Build history of the part. All positions in model axes, mm. Face numbers are marked on the shaded views. A direction names the side the tool comes from. Give positions to 0.01 mm unless a question says otherwise; leave off trailing zeros. Write each loop counter-clockwise with the first axis right and the second up, starting at its lowest first coordinate (ties: lowest second). Pieces come first, ordered by that corner, then holes. Notation, with made-up numbers: (79.25, 2.25) -> (84.25, 2.25) arc R14 ccw to (84.25, 12.25) -> close; hole circle Ø3 at (15, 44.5). An arc over 180 degrees is marked (long way). Put each result on its own line as item: value.
from build123d import *

# Parameters (mm, degrees)
BOSS_EXTRUDE1_DEPTH      = 7
SKETCH2_R                = 2.05
CUT_EXTRUDE1_DEPTH       = 210.034905978
CUT_EXTRUDE2_DEPTH       = 4
BOSS_EXTRUDE8_DEPTH      = 7
BOSS_EXTRUDE8_DEPTH_BACK = 1
BOSS_EXTRUDE9_DEPTH      = 8
SKETCH22_R               = 2
CUT_EXTRUDE3_DEPTH       = 211.072825271
CUT_EXTRUDE4_DEPTH       = 4
CHAMFER1_SIZE            = 0.5
CHAMFER2_SIZE            = 0.5
CHAMFER3_SIZE            = 4


with BuildPart() as part:
    # Sketch1 → Boss-Extrude1 (new body)
    with BuildSketch(Plane.XY):
        Polygon((-86.168640192, 66.168375393), (-46.796854981, 26.9381166), (-46.864915159, 16.542640687), (-68.155605804, 16.542640687), (-75.083809034, 4.542640687), (-88.767010414, 4.542640687), (-95.695213644, 16.542640687), (-127.7, 16.542640687), (-127.7, 21.829570993), (-140.170429007, 34.3), (-155.457359313, 34.3), (-155.457359313, 76.089816153), (-167.457359313, 83.018019384), (-167.457359313, 96.701220763), (-155.457359313, 103.629423994), (-155.457359313, 124.918472329), (-145.062341245, 124.850415149), (-105.649268389, 85.614252867), (-92.265224659, 89.200496576), (-82.589740175, 79.525012092), align=None)
    extrude(amount=-BOSS_EXTRUDE1_DEPTH)

    # Sketch2 → Cut-Extrude1 (cut, through all)
    with BuildSketch(Plane(origin=(0, 0, -7), x_dir=(-1, 0, 0), z_dir=(0, 0, -1))):
        with Locations((82.1403802, 10.392640687)):
            Circle(SKETCH2_R)
        with Locations((91.564057064, 80.226179394)):
            Circle(SKETCH2_R)
        with Locations((161.607359313, 89.8596198)):
            Circle(SKETCH2_R)
    extrude(amount=-CUT_EXTRUDE1_DEPTH, mode=Mode.SUBTRACT)

    # Sketch3 → Cut-Extrude2 (cut)
    with BuildSketch(Plane.XY):
        Polygon((-158.61957167, 88.1346198), (-158.61957167, 91.5846198), (-161.607359313, 93.3096198), (-164.595146956, 91.5846198), (-164.595146956, 88.1346198), (-161.607359313, 86.4096198), align=None)
        Polygon((-88.231612963, 81.1191051), (-90.671131358, 83.558623495), (-94.003575459, 82.665697789), (-94.896501165, 79.333253689), (-92.456982769, 76.893735294), (-89.124538669, 77.786660999), align=None)
        Polygon((-80.4153802, 7.404853044), (-78.6903802, 10.392640687), (-80.4153802, 13.38042833), (-83.8653802, 13.38042833), (-85.5903802, 10.392640687), (-83.8653802, 7.404853044), align=None)
    extrude(amount=-CUT_EXTRUDE2_DEPTH, mode=Mode.SUBTRACT)

    # Sketch19 → Boss-Extrude8 (add, two sides: drawn at the far end of the back side and taken through both)
    with BuildSketch(Plane(origin=(0, 0, -7), x_dir=(-1, 0, 0), z_dir=(0, 0, -1)).offset(-BOSS_EXTRUDE8_DEPTH_BACK)):
        Polygon((46.864915159, 16.542640687), (46.796854981, 26.9381166), (145.062341245, 124.850415149), (155.457359313, 124.918472329), (155.457359313, 34.3), (140.170429007, 34.3), (127.7, 21.829570993), (127.7, 16.542640687), align=None)
    extrude(amount=BOSS_EXTRUDE8_DEPTH + BOSS_EXTRUDE8_DEPTH_BACK)

    # Sketch20 → Boss-Extrude9 (add)
    with BuildSketch(Plane(origin=(0, 0, -14), x_dir=(-1, 0, 0), z_dir=(0, 0, -1))):
        Polygon((127.7, 16.542640687), (107.164334943, 16.542640687), (71.827840432, 51.879135198), (119.997668017, 99.875829855), (155.457359313, 64.416138559), (155.457359313, 34.3), (140.170429007, 34.3), (127.7, 21.829570993), align=None)
    extrude(amount=BOSS_EXTRUDE9_DEPTH)

    # Sketch22 → Cut-Extrude3 (cut, through all)
    with BuildSketch(Plane(origin=(0, 0, -22), x_dir=(-1, 0, 0), z_dir=(0, 0, -1))):
        with Locations((100.752632712, 46.288866697)):
            Circle(SKETCH22_R)
        with Locations((125.501370054, 71.037604039)):
            Circle(SKETCH22_R)
    extrude(amount=-CUT_EXTRUDE3_DEPTH, mode=Mode.SUBTRACT)

    # Sketch23 → Cut-Extrude4 (cut)
    with BuildSketch(Plane.XY):
        Polygon((-125.501370054, 74.487604039), (-128.489157697, 72.762604039), (-128.489157697, 69.312604039), (-125.501370054, 67.587604039), (-122.513582411, 69.312604039), (-122.513582411, 72.762604039), align=None)
        Polygon((-104.202632712, 46.288866697), (-102.477632712, 43.301079054), (-99.027632712, 43.301079054), (-97.302632712, 46.288866697), (-99.027632712, 49.27665434), (-102.477632712, 49.27665434), align=None)
    extrude(amount=-CUT_EXTRUDE4_DEPTH, mode=Mode.SUBTRACT)

    # Chamfer1
    chamfer1_edges = [part.edges().sort_by_distance(p)[0] for p in [
        (-160.113465491, 87.2721198, 0),
        (-158.61957167, 89.8596198, 0),
        (-160.113465491, 92.4471198, 0),
        (-163.101253134, 92.4471198, 0),
        (-164.595146956, 89.8596198, 0),
        (-163.101253134, 87.2721198, 0),
        (-88.678075816, 79.45288305, 0),
        (-89.451372161, 82.338864297, 0),
        (-92.337353409, 83.112160642, 0),
        (-94.450038312, 80.999475739, 0),
        (-93.676741967, 78.113494491, 0),
        (-90.790760719, 77.340198146, 0),
        (-82.1403802, 7.404853044, 0),
        (-79.5528802, 8.898746866, 0),
        (-79.5528802, 11.886534509, 0),
        (-82.1403802, 13.38042833, 0),
        (-84.7278802, 11.886534509, 0),
        (-84.7278802, 8.898746866, 0),
    ]]
    chamfer(chamfer1_edges, length=CHAMFER1_SIZE)

    # Chamfer2
    chamfer2_edges = [part.edges().sort_by_distance(p)[0] for p in [
        (-124.007476232, 73.625104039, 0),
        (-126.995263875, 73.625104039, 0),
        (-128.489157697, 71.037604039, 0),
        (-126.995263875, 68.450104039, 0),
        (-124.007476232, 68.450104039, 0),
        (-122.513582411, 71.037604039, 0),
        (-103.340132712, 47.782760519, 0),
        (-103.340132712, 44.794972876, 0),
        (-100.752632712, 43.301079054, 0),
        (-98.165132712, 44.794972876, 0),
        (-98.165132712, 47.782760519, 0),
        (-100.752632712, 49.27665434, 0),
    ]]
    chamfer(chamfer2_edges, length=CHAMFER2_SIZE)

    # Chamfer3
    chamfer3_edges = [part.edges().sort_by_distance(p)[0] for p in [
        (-137.727513665, 82.145984207, -14),
        (-89.496087688, 34.210887943, -14),
    ]]
    chamfer(chamfer3_edges, length=CHAMFER3_SIZE)


solid = part.part
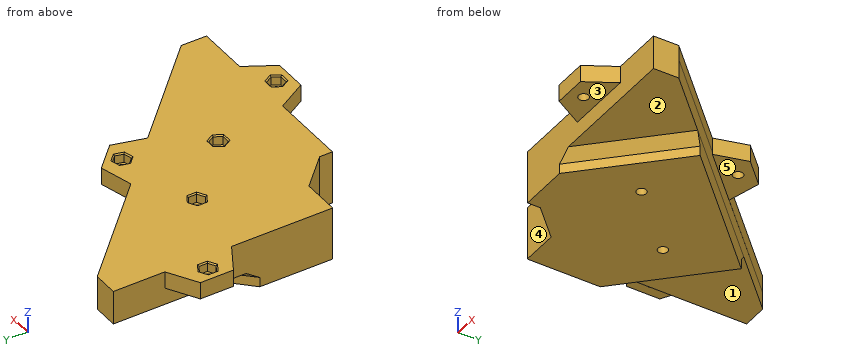
1) Slice it at A-A (z = -9.75). Write the cut outline in (x, y), plus the area to 3 significant figures.
Filled sheet:
outline: (-155.46, 34.3) -> (-140.17, 34.3) -> (-127.7, 21.83) -> (-127.7, 16.54) -> (-46.86, 16.54) -> (-46.8, 26.94) -> (-145.06, 124.85) -> (-155.46, 124.92) -> close; hole circle Ø4 at (-125.5, 71.04); hole circle Ø4 at (-100.75, 46.29)
area: 6,520 mm2
2) Pin check, flat tips, straight feed: pin 1 (3.5 mm diameter, centred on x = -82.5, y = 8, fed in from -Z); pin 2 (3 mm diameter, centred on x = -81.5, z = -2, fed in from +Y); pin 3 (2 mm diameter, centred on x = -99.5, z = -4, fed in from +Y). Stop position of each tip, or through.
Filled sheet:
pin 1: z = -7
pin 2: y = 79.94
pin 3: y = 87.53
3) Wall check: L1, parallel to Y at x = -101, z = -3.75; L2, parallel to Y at x = -126, z = -14.5; L3, parallel to Y at x = -149.5, z = -13.25. Give the ranges that are in metal, low to high.
Filled sheet:
L1: 16.54 to 43.3, 49.28 to 86.86
L2: 16.54 to 69.1, 72.97 to 98.82
L3: 34.3 to 124.88
4) Tool access for the marked faces 1, 2, 3, 4 and 5: list every direction of +Z, -Z, +X, -X, +Y, -Y with a clear straight run to the whole face (end or side of a thin tool).
Filled sheet:
face 1: -Z, -X, +Y
face 2: -Z, +X, -Y
face 3: -Z, +X, -X, -Y
face 4: +Z, -Z, -X, -Y
face 5: -Z, +X, +Y
